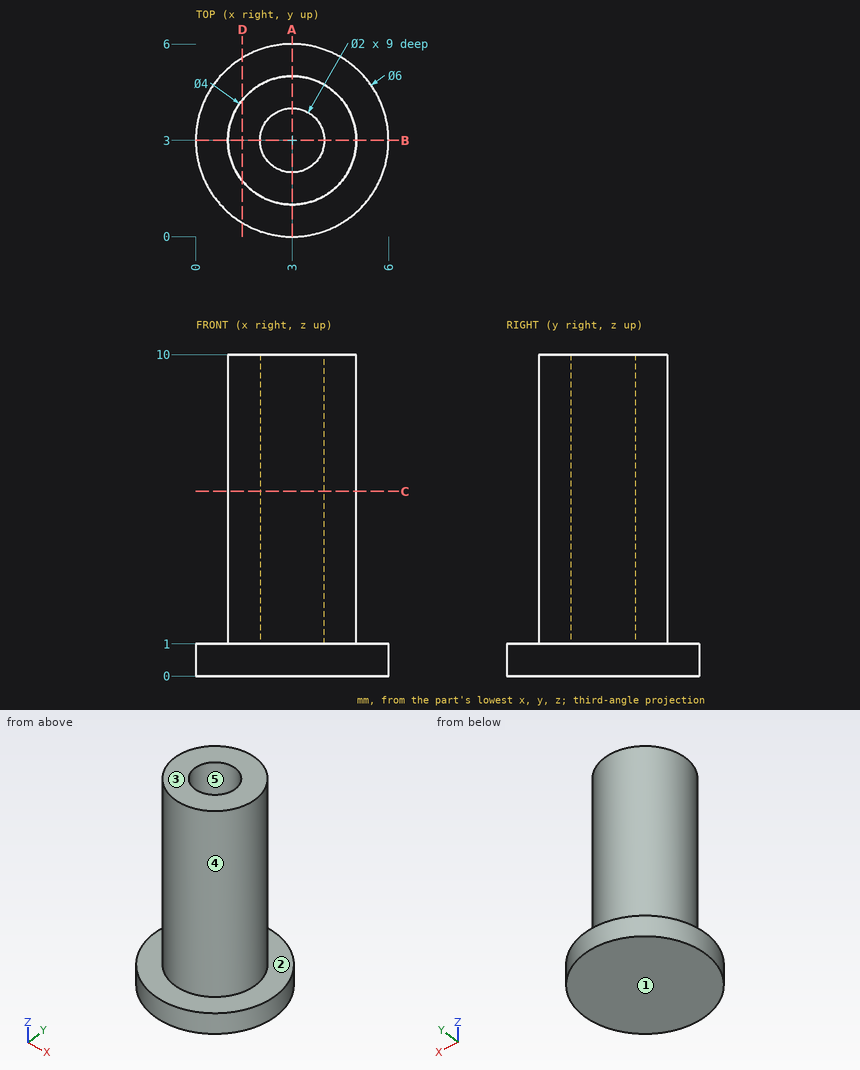
The drawing under review shows one solid part. Ordinate dimensions are in mm from its lowest x, y, z. A direction names the side the tool comes from. Coordinates: 2 decimals unless noted, no trailing zeros. Order: outer loops, then holes, each group sorted by start corner. A loop starts at its lowest first (then second) coordinate and runs counter-clockwise, first axis right, second up. Notation, with made-up numbers: (-11.75, 63.5) -> (22.25, 63.5) arc R29 cw to (22.25, 97.5) -> close; hole circle Ø9 at (60.25, 67). An arc over 180 degrees is marked (long way). Answer in a Markdown table with one row per item. Add a question column.
Item 1: Machinability: for the marked faces 1 and 2, which of the approach directions +Z, -Z, +X, -X, +Y, -Y give a long, thin tool a straight path to every point of the face, cutting with its end or side? Answer none if there is none.
Item 2: Mouldability with a two-part tool opening along X and no side actions: class the marked faces 3, 4 and 5 as +X half, -X half, draft (parallel to the pull), parting line (faces both ways), or undercut.
Item 3: We need section A-A on x = 3. Write out the cut boundary in (y, z).
Item 4: Clearance check with flat-ended pins moving along their axes: pin 1 (2.5 mm diameter, centred on x = 3, y = 3, fed in from +Z); pin 2 (2 mm diameter, centred on x = 1.5, z = 6.5, fed in from +Y); pin 3 (0.6 mm diameter, centred on x = 2.5, y = 3, fed in from +Z); pin 4 (3 mm diameter, centred on y = 5.5, z = 7.5, fed in from -X). State where each tip first meets the part, or that it passes through.
Item 5: To check wall thickness, follow probe 1 along Y at (x, z) = (3, 5.5); probe 2 along Z at (x, y) = (4.35, 0.9). State the ranges of each line that lie inside material, in increasing order.
Item 6: We need section C-C on z = 5.75. Write out the cut boundary in (x, y).
Item 7: We need section D-D on x = 1.45. Write out the cut boundary in (y, z).
Final values:
| question | item | result |
|---|---|---|
| 1 | face 1 | -Z, +X, -X, +Y, -Y |
| 1 | face 2 | +Z |
| 2 | face 3 | draft |
| 2 | face 4 | parting line |
| 2 | face 5 | undercut |
| 3 | outline | (0, 0) -> (6, 0) -> (6, 1) -> (5, 1) -> (5, 10) -> (4, 10) -> (4, 1) -> (2, 1) -> (2, 10) -> (1, 10) -> (1, 1) -> (0, 1) -> close |
| 4 | pin 1 | stops at z = 10 |
| 4 | pin 2 | stops at y = 4.94 |
| 4 | pin 3 | stops at z = 1 |
| 4 | pin 4 | stops at x = 1.27 |
| 5 | probe 1 | y = 1 to 2, 4 to 5 |
| 5 | probe 2 | z = 0 to 1 |
| 6 | outline | circle Ø4 at (3, 3); hole circle Ø2 at (3, 3) |
| 7 | outline | (0.43, 0) -> (5.57, 0) -> (5.57, 1) -> (4.26, 1) -> (4.26, 10) -> (1.74, 10) -> (1.74, 1) -> (0.43, 1) -> close |
